Autodesk Inventor part; units mm, degrees
ref_plane "YZ Plane" through (0, 0, 0) normal (1, 0, 0) x (0, 1, 0)
ref_plane "XZ Plane" through (0, 0, 0) normal (0, 1, 0) x (-1, 0, 0)
ref_plane "XY Plane" through (0, 0, 0) normal (0, 0, 1) x (1, 0, 0)
sketch "Sketch1" plane through (0, 0, 0) normal (0, 0, 1) x (1, 0, 0)
  line L0 (0, 0) -> (50.8, 0)
  line L1 (50.8, 0) -> (50.8, 25.4)
  line L2 (50.8, 25.4) -> (0, 25.4)
  line L3 (0, 25.4) -> (0, 0)
  line L4 (1.5875, 1.5875) -> (49.2125, 1.5875)
  line L5 (49.2125, 1.5875) -> (49.2125, 23.8125)
  line L6 (49.2125, 23.8125) -> (1.5875, 23.8125)
  line L7 (1.5875, 23.8125) -> (1.5875, 1.5875)
  dimension "d0" = 50.8
  dimension "d1" = 25.4
  dimension "d2" = 1.5875
extrude "Extrusion1" add sketch "Sketch1" along normal mid plane 615.95
chamfer "Chamfer1" distance 25.4 angle 45 2 edges at (25.4, 25.4, 307.975) (25.4, 25.4, -307.975)
properties part number "FRA_006_FrontMainRail" material "Aluminum 6061"
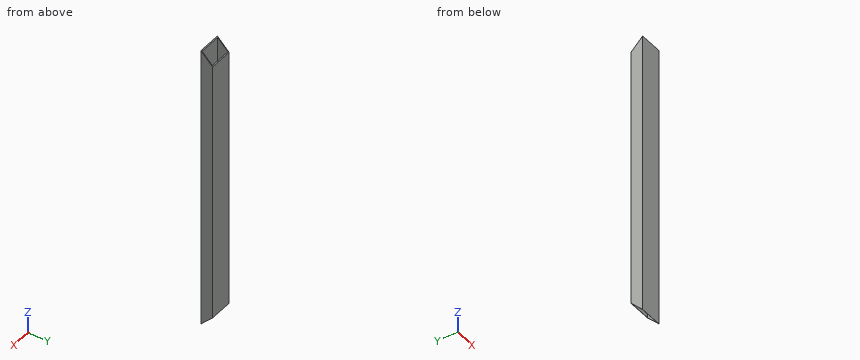
Design review of the part built by this model. Coordinates are the model's own, in mm. Give positions to 0.01 mm unless a question says otherwise; leave off trailing zeros. Loops run counter-clockwise (first coordinate to the right, second up) from the corner with the lowest first, then second, coordinate; pieces in that order, holes last. Notation, with made-up numbers: M -23.5,84 L -2.5,84 A9 cw -2.5,91 Z; hole C 45,74.5 d8. An arc over 180 degrees is marked long. Return JSON: item names as keys, results as strings. Group by question number.
Item 1: For probe 1 along Y at (x, z) = (48, 173.5); probe 2 along X at (y, z) = (10.25, 268); probe 3 along Z at (x, y) = (44.5, 1.5) (3 decimals), list the stretches that pass through material, from the lowest coordinate up.
Item 2: We need section C-C (z = -29.5). Give the boundary of the cut face in (x, y), and give its area (3 significant figures).
Item 3: We need section A-A (x = 27). Give the boundary of the cut face in (y, z) (1 decimal).
Item 4: Insertion check: pin 1 Ø12 at (x, y) = (6, 6.5) entering from +Z (3 decimals). The pin has a flat end and moves straight along its axis. Give the tip position at first contact, or say it passes through.
Item 5: We need section B-B (y = 10.25). Give the boundary of the cut face in (x, z) (1 decimal), and give its area (3 significant figures).
Output:
{
 "1": {"probe 1": "y = 0 to 1.59, 23.81 to 25.4", "probe 2": "x = 0 to 1.59, 49.21 to 50.8", "probe 3": "z = -306.475 to 306.475"},
 "2": {"outline": "M 0,0 L 50.8,0 L 50.8,25.4 L 0,25.4 Z; hole M 1.59,1.59 L 49.21,1.59 L 49.21,23.81 L 1.59,23.81 Z", "area": "232 mm^2"},
 "3": {"outline": "M 0,-308 L 1.6,-306.4 L 1.6,306.4 L 0,308 Z; M 23.8,-284.2 L 25.4,-282.6 L 25.4,282.6 L 23.8,284.2 Z"},
 "4": {"pin 1": "stops at z = 307.475"},
 "5": {"outline": "M 0,-297.7 L 1.6,-297.7 L 1.6,297.7 L 0,297.7 Z; M 49.2,-297.7 L 50.8,-297.7 L 50.8,297.7 L 49.2,297.7 Z", "area": "1,890 mm^2"}
}
